Read the model definition and answer for the solid it produces. Units are mm, in the model's axes. Face numbers are marked on the shaded views. A direction names the side the tool comes from. Coordinates: 2 decimals unless noted, no trailing zeros. Order: outer loops, then holes, each group sorted by start corner. A loop starts at its lowest first (then second) coordinate and runs counter-clockwise, first axis right, second up. Notation, with made-up numbers: (-38.75, -12) -> (-15.75, -12) arc R21 ccw to (-15.75, 21) -> close; hole circle Ø11 at (-7, 50.25). An arc over 180 degrees is marked (long way). Answer in a Markdown table with one row per item.
from build123d import *

# Parameters (mm, degrees)
SKETCH2_R                       = 3
BOSS_EXTRUDE3_DEPTH             = 18.5
SKETCH3_R                       = 6
BOSS_EXTRUDE5_DEPTH             = 0.5
SKETCH5_R                       = 24.9
BOSS_EXTRUDE6_DEPTH             = 65.5
SKETCH6_R                       = 4
BOSS_EXTRUDE7_DEPTH             = 32
CHAMFER1_SIZE                   = 3
CHAMFER1_SIZE2                  = 12
CHAMFER2_SIZE                   = 10
SKETCH7_R                       = 14.9
BOSS_EXTRUDE8_DEPTH             = 5
M4X0_7_TAPPED_HOLE1_D           = 3.3
M4X0_7_TAPPED_HOLE1_DEPTH       = 10.508579979
M4X0_7_TAPPED_HOLE1_CSINK_D     = 4.05
M4X0_7_TAPPED_HOLE1_CSINK_ANGLE = 90
M4X0_7_TAPPED_HOLE1_TIP         = 0.991420021


with BuildPart() as part:
    # Sketch2 → Boss-Extrude3 (new body)
    with BuildSketch(Plane(origin=(0, 0, 0), x_dir=(1, 0, 0), z_dir=(0, 1, 0))):
        with Locations(Location((0, 0, 0), (0, 0, 270))):
            Circle(SKETCH2_R)
    extrude(amount=BOSS_EXTRUDE3_DEPTH)

    # Sketch3 → Boss-Extrude5 (add)
    with BuildSketch(Plane(origin=(0, 18.5, 0), x_dir=(1, 0, 0), z_dir=(0, 1, 0))):
        with Locations(Location((0, 0, 0), (0, 0, 270))):
            Circle(SKETCH3_R)
    extrude(amount=BOSS_EXTRUDE5_DEPTH)

    # Sketch5 → Boss-Extrude6 (add)
    with BuildSketch(Plane(origin=(0, 19, 0), x_dir=(1, 0, 0), z_dir=(0, 1, 0))):
        with Locations(Location((0, 0, 0), (0, 0, 270))):
            Circle(SKETCH5_R)
    extrude(amount=BOSS_EXTRUDE6_DEPTH)

    # Sketch6 → Boss-Extrude7 (add)
    with BuildSketch(Plane(origin=(0, 84.5, 0), x_dir=(1, 0, 0), z_dir=(0, 1, 0))):
        with Locations(Location((0, 0, 0), (0, 0, 270))):
            Circle(SKETCH6_R)
    extrude(amount=BOSS_EXTRUDE7_DEPTH)

    # Chamfer1
    chamfer1_edges = [part.edges().sort_by_distance(p)[0] for p in [
        (0, 19, -24.9),
    ]]
    chamfer1_side = [part.faces().sort_by_distance(p)[0] for p in [
        (0, 19, -24.195721646),
    ]]
    chamfer(chamfer1_edges, length=CHAMFER1_SIZE, length2=CHAMFER1_SIZE2, reference=chamfer1_side[0])

    # Chamfer2
    chamfer2_edges = [part.edges().sort_by_distance(p)[0] for p in [
        (0, 84.5, -24.9),
    ]]
    chamfer(chamfer2_edges, length=CHAMFER2_SIZE)

    # Sketch7 → Boss-Extrude8 (add)
    with BuildSketch(Plane(origin=(0, 84.5, 0), x_dir=(1, 0, 0), z_dir=(0, 1, 0))):
        with Locations(Location((0, 0, 0), (0, 0, 270))):
            Circle(SKETCH7_R)
    extrude(amount=BOSS_EXTRUDE8_DEPTH)

    # M4x0.7 Tapped Hole1
    with Locations(Plane(origin=(0, 19, 0), x_dir=(-1, 0, 0), z_dir=(0, -1, 0))):
        with Locations((-10.606601718, 10.606601718), (10.606601718, -10.606601718), (10.606601718, 10.606601718), (-10.606601718, -10.606601718)):
            CounterSinkHole(M4X0_7_TAPPED_HOLE1_D / 2, M4X0_7_TAPPED_HOLE1_CSINK_D / 2, depth=M4X0_7_TAPPED_HOLE1_DEPTH, counter_sink_angle=M4X0_7_TAPPED_HOLE1_CSINK_ANGLE)
            with Locations((0, 0, -(M4X0_7_TAPPED_HOLE1_DEPTH + M4X0_7_TAPPED_HOLE1_TIP / 2))):  # 118° drill point
                Cone(0, M4X0_7_TAPPED_HOLE1_D / 2, M4X0_7_TAPPED_HOLE1_TIP, mode=Mode.SUBTRACT)


solid = part.part
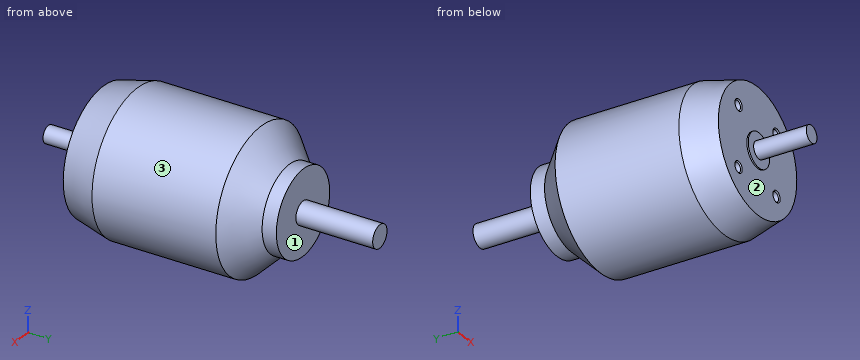
Q1. The part is cut by section C-C (y = 107.5). Write down the section's boundary in (x, z).
Outcome:
| item | result |
|---|---|
| outline | circle Ø8 at (0, 0) |
Q2. Given pin 1 (4 mm diameter, centred on x = 14, z = 13.5, fed in from -Y); pin 2 (13 mm diameter, centred on x = -3.5, z = -2.5, fed in from -Y); pin 3 (2 mm diameter, centred on x = -10.61, z = -10.61, fed in from -Y); pin 4 (2 mm diameter, centred on x = 10.61, z = 10.61, fed in from +Y), each flat-ended and moving along its own axis, determine where each tip first touches the part or whether it passes through.
Outcome:
| item | result |
|---|---|
| pin 1 | y = 19 |
| pin 2 | y = 0 |
| pin 3 | y = 29.9 |
| pin 4 | y = 89.5 |
Q3. For the marked faces 1, 2 and 3, determine the directions among +Z, -Z, +X, -X, +Y, -Y from which every point of the face is accessible in a straight line to the end or side of a thin tool.
Outcome:
| item | result |
|---|---|
| face 1 | +Y |
| face 2 | -Y |
| face 3 | +Y, -Y |
Q4. The part is cut by section B-B (x = 0). Write down the section's boundary in (y, z), then the cut area to 3 significant figures.
Outcome:
| item | result |
|---|---|
| outline | (0, -3) -> (18.5, -3) -> (18.5, -6) -> (19, -6) -> (19, -21.9) -> (31, -24.9) -> (74.5, -24.9) -> (84.5, -14.9) -> (89.5, -14.9) -> (89.5, -4) -> (116.5, -4) -> (116.5, 4) -> (89.5, 4) -> (89.5, 14.9) -> (84.5, 14.9) -> (74.5, 24.9) -> (31, 24.9) -> (19, 21.9) -> (19, 6) -> (18.5, 6) -> (18.5, 3) -> (0, 3) -> close |
| area | 3,610 mm² |
Q5. The part is cut by section D-D (y = 9). Write down the section's boundary in (x, z), then the cut area to 3 significant figures.
Outcome:
| item | result |
|---|---|
| outline | circle Ø6 at (0, 0) |
| area | 28.3 mm² |
Q6. The part is cut by section A-A (z = 0). Write down the section's boundary in (x, y), then the cut area to 3 significant figures.
Outcome:
| item | result |
|---|---|
| outline | (-24.9, 31) -> (-21.9, 19) -> (-6, 19) -> (-6, 18.5) -> (-3, 18.5) -> (-3, 0) -> (3, 0) -> (3, 18.5) -> (6, 18.5) -> (6, 19) -> (21.9, 19) -> (24.9, 31) -> (24.9, 74.5) -> (14.9, 84.5) -> (14.9, 89.5) -> (4, 89.5) -> (4, 116.5) -> (-4, 116.5) -> (-4, 89.5) -> (-14.9, 89.5) -> (-14.9, 84.5) -> (-24.9, 74.5) -> close |
| area | 3,610 mm² |
Q7. Consider line 1 (Y direction, x = 7, z = 6); line 2 (Z direction, x = -11, y = 22.5); line 3 (Z direction, x = -3.5, y = 34). Determine where each line is inside the solid, lowest interval first.
Outcome:
| item | result |
|---|---|
| line 1 | 19 to 89.5 |
| line 2 | -19.94 to -12.21, -9 to 9, 12.21 to 19.94 |
| line 3 | -24.65 to 24.65 |
